The model under review builds one solid part; all positions refer to its coordinate system, in mm. Round coordinates to 2 decimals unless told otherwise and drop trailing zeros. Write each loop counter-clockwise with the first axis right and the second up, starting at its lowest first coordinate (ties: lowest second). Pieces come first, ordered by that corner, then holes. Notation, with made-up numbers: (2, 29) -> (56, 29) arc R10 ccw to (56, 48) -> close; hole circle Ø3 at (65.25, 33.25). An arc over 180 degrees is marked (long way). Use CSV: the item, a comma, the result in double quotes. Start each with the question number.
1) Take a section at D-D, the plane x = 40. Give the boundary of the cut face in (y, z).
2) Take a section at A-A, the plane x = 54. Give the boundary of the cut face in (y, z), then the cut area to 3 significant figures.
3) Take a section at C-C, the plane z = 0.4. Give the boundary of the cut face in (x, y), then the cut area to 3 significant figures.
4) Wall thickness on probe 1 along X at (y, z) = (6.5, 0.4); probe 2 along X at (y, z) = (12.25, 0.4); probe 3 along X at (y, z) = (3, 0.25): over which ranges is each line inside the solid? List them lowest first. Write a range as [from, to].
5) Take a section at B-B, the plane y = 10.75. Give the boundary of the cut face in (x, z).
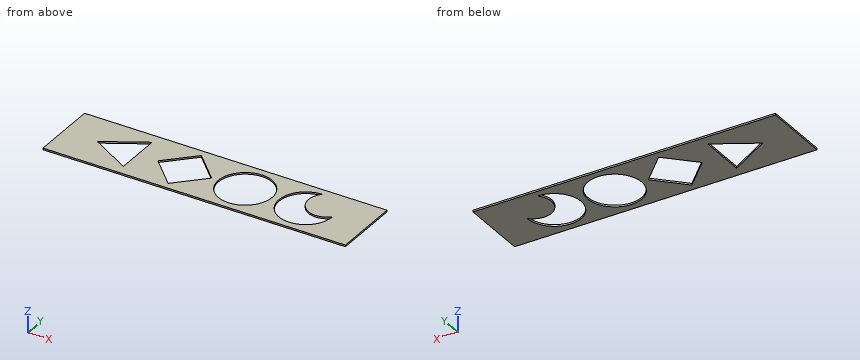
from build123d import *

# Parameters (mm, degrees)
SKETCH_W  = 90
SKETCH_H  = 20
SKETCH_R  = 8
PAD_DEPTH = 0.5


with BuildPart() as part:
    # Sketch → Pad (new body)
    with BuildSketch(Plane.XY):
        with Locations((45, 10)):
            Rectangle(SKETCH_W, SKETCH_H)
        with Locations((54, 10)):
            Circle(SKETCH_R, mode=Mode.SUBTRACT)
        Polygon((44, 10), (36, 18), (28, 10), (36, 2), align=None, mode=Mode.SUBTRACT)
        with BuildLine():
            ThreePointArc((72, 18), (66.343146, 4.343146), (80, 10))
            ThreePointArc((72, 18), (72, 10), (80, 10))
        make_face(mode=Mode.SUBTRACT)
        Polygon((22, 3.071824), (22, 16.92823), (10, 10.000027), align=None, mode=Mode.SUBTRACT)
    extrude(amount=PAD_DEPTH)


solid = part.part
Values found:
1,outline,"(0, 0) -> (6, 0) -> (6, 0.5) -> (0, 0.5) -> close; (14, 0) -> (20, 0) -> (20, 0.5) -> (14, 0.5) -> close"
2,outline,"(0, 0) -> (2, 0) -> (2, 0.5) -> (0, 0.5) -> close; (18, 0) -> (20, 0) -> (20, 0.5) -> (18, 0.5) -> close"
2,area,"2.00 mm²"
3,outline,"(0, 0) -> (90, 0) -> (90, 20) -> (0, 20) -> close; hole (10, 10) -> (22, 3.07) -> (22, 16.93) -> close; hole (28, 10) -> (36, 2) -> (44, 10) -> (36, 18) -> close; hole circle Ø16 at (54, 10); hole (72, 18) arc R8 ccw (long way) to (80, 10) arc R5.66 cw to start"
3,area,"1,260 mm²"
4,probe 1,"[0, 16.06], [22, 31.5], [40.5, 46.81], [61.19, 64.81], [79.19, 90]"
4,probe 2,"[0, 13.9], [22, 30.25], [41.75, 46.32], [61.68, 64.32], [70.62, 90]"
4,probe 3,"[0, 35], [37, 50.13], [57.87, 68.13], [75.87, 90]"
5,outline,"(0, 0) -> (11.3, 0) -> (11.3, 0.5) -> (0, 0.5) -> close; (22, 0) -> (28.75, 0) -> (28.75, 0.5) -> (22, 0.5) -> close; (43.25, 0) -> (46.04, 0) -> (46.04, 0.5) -> (43.25, 0.5) -> close; (61.96, 0) -> (64.04, 0) -> (64.04, 0.5) -> (61.96, 0.5) -> close; (71.37, 0) -> (90, 0) -> (90, 0.5) -> (71.37, 0.5) -> close"
